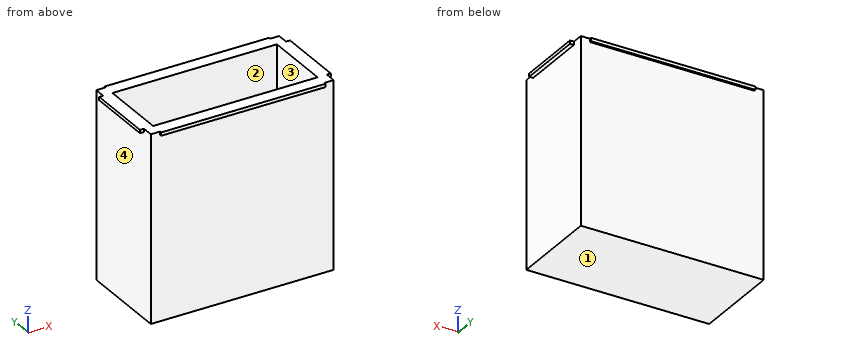
from build123d import *

# Parameters (mm, degrees)
SKETCH1_W           = 13.9
SKETCH1_H           = 6.85
BOSS_EXTRUDE1_DEPTH = 14.15
SKETCH2_W           = 12.5
SKETCH2_H           = 5.12
CUT_EXTRUDE1_DEPTH  = 13
SKETCH4_W           = 12.5
SKETCH4_H           = 0.25
BOSS_EXTRUDE2_DEPTH = 0.135
SKETCH5_W           = 0.25
SKETCH5_H           = 5.12
BOSS_EXTRUDE3_DEPTH = 0.3


with BuildPart() as part:
    # Sketch1 → Boss-Extrude1 (new body)
    with BuildSketch(Plane.XY):
        Rectangle(SKETCH1_W, SKETCH1_H)
    extrude(amount=BOSS_EXTRUDE1_DEPTH)

    # Sketch2 → Cut-Extrude1 (cut)
    with BuildSketch(Plane.XY.offset(14.15)):
        Rectangle(SKETCH2_W, SKETCH2_H)
    extrude(amount=-CUT_EXTRUDE1_DEPTH, mode=Mode.SUBTRACT)

    # Sketch4 → Boss-Extrude2 (add)
    with BuildSketch(Plane(origin=(0, 3.425, 0), x_dir=(1, 0, 0), z_dir=(0, 1, 0))):
        with Locations((0, -14.025)):
            Rectangle(SKETCH4_W, SKETCH4_H)
    boss_extrude2 = extrude(amount=BOSS_EXTRUDE2_DEPTH)

    # Mirror1: Boss-Extrude2 across plane
    add(boss_extrude2.mirror(Plane.ZX))

    # Sketch5 → Boss-Extrude3 (add)
    with BuildSketch(Plane(origin=(6.95, 0, 0), x_dir=(0, 0, -1), z_dir=(1, 0, 0))):
        with Locations((-14.025, 0)):
            Rectangle(SKETCH5_W, SKETCH5_H)
    boss_extrude3 = extrude(amount=BOSS_EXTRUDE3_DEPTH)

    # Mirror2: Boss-Extrude3 across plane
    add(boss_extrude3.mirror(Plane(origin=(0, 0, 0), x_dir=(0, 0, 1), z_dir=(1, 0, 0))))


solid = part.part
Verification items for the finished model (mm, model axes). Face numbers are marked on the shaded views. A direction names the side the tool comes from. Coordinates: 2 decimals unless noted, no trailing zeros. Write each loop counter-clockwise with the first axis right and the second up, starting at its lowest first coordinate (ties: lowest second). Pieces come first, ordered by that corner, then holes. Notation, with made-up numbers: (43, 25.25) -> (97, 25.25) arc R31 ccw to (97, 60.25) -> close; hole circle Ø10 at (73.25, -5). An arc over 180 degrees is marked (long way). One line per item, written item: value. Start each with the question number.
Q1. Cross-section at B-B on y = 0.25. Enter the section's corners in (x, z), and give its area (3 significant figures).
Q2. Access from +Z, -Z, +X, -X, +Y, -Y to the whole of each face (thin tool, end or side, straight path). Record for the marked faces 1 and 2.
Q3. Go/stop test with flat-tipped pins: P1, Ø4, axis at x = -1, z = 4.5, coming from the -Y side (3 decimals); P2, Ø1, axis at y = 1.5, z = 2.5, coming from the -X side; P3, Ø4, axis at x = 3.5, z = 10, coming from the +Y side (3 decimals). Record where each tip stops, or that it passes through.
Q4. Cross-section at A-A on z = 2. Enter the section's corners in (x, y) (3 decimals).
Q5. Mould release check, pull along Y, two halves, no side actions. Record for the marked faces 3 and 4: pulls with the +Y half, pulls with the -Y half, needs draft (parallel to the pull), parting line crosses it, or undercut.
Q6. Thickness scan on L1, parallel to X at y = -2, z = 8.5; L2, parallel to Y at x = 6, z = 12.5 (3 decimals); L3, parallel to X at y = 3, z = 10.5. Record the ranges inside material, lowest first. Write a range as from..to.
Q7. Cross-section at C-C on x = -2. Enter the section's corners in (y, z) (3 decimals), and give its area (3 significant figures).
Checked values:
1. outline: (-7.25, 13.9) -> (-6.95, 13.9) -> (-6.95, 0) -> (6.95, 0) -> (6.95, 13.9) -> (7.25, 13.9) -> (7.25, 14.15) -> (6.25, 14.15) -> (6.25, 1.15) -> (-6.25, 1.15) -> (-6.25, 14.15) -> (-7.25, 14.15) -> close
1. area: 34.3 mm²
2. face 1: -Z, +X, -X, +Y, -Y
2. face 2: +Z
3. P1: stops at y = -3.425
3. P2: stops at x = -6.95
3. P3: stops at y = 3.425
4. outline: (-6.95, -3.425) -> (6.95, -3.425) -> (6.95, 3.425) -> (-6.95, 3.425) -> close; hole (-6.25, -2.56) -> (6.25, -2.56) -> (6.25, 2.56) -> (-6.25, 2.56) -> close
5. face 3: undercut
5. face 4: needs draft
6. L1: x = -6.95..-6.25, 6.25..6.95
6. L2: y = -3.425..-2.56, 2.56..3.425
6. L3: x = -6.95..6.95
7. outline: (-3.56, 13.9) -> (-3.425, 13.9) -> (-3.425, 0) -> (3.425, 0) -> (3.425, 13.9) -> (3.56, 13.9) -> (3.56, 14.15) -> (2.56, 14.15) -> (2.56, 1.15) -> (-2.56, 1.15) -> (-2.56, 14.15) -> (-3.56, 14.15) -> close
7. area: 30.4 mm²
